Autodesk Inventor part; units mm, degrees
ref_plane "Work Plane1" through (150, 0, 0) normal (1, 0, 0) x (0, 0, -1)
ref_plane "Work Plane2" through (100.659, 0, -74) normal (0, 0, -1) x (-1, 0, 0)
ref_plane "Work Plane3" through (150, 0, 0) normal (1, 0, 0) x (0, 0, -1)
sketch "Sketch1" plane through (0, 0, 0) normal (0, 1, 0) x (-1, 0, 0)
  line L0 (0, 0) -> (-300, 0)
  line L1 (-300, 0) -> (-300, -148)
  line L2 (-300, -148) -> (0, -148)
  line L3 (0, -148) -> (0, 0)
  dimension "d0" = 300
  dimension "d1" = 148
extrude "Extrusion1" add sketch "Sketch1" along normal blind 4
sketch "Sketch2" plane through (0, 0, 0) normal (0, -1, 0) x (1, 0, 0)
  line L0 (0, -74) -> (300, -74) construction
  line L1 (150, 0) -> (150, -148) construction
sketch "Sketch3" plane through (0, 0, 0) normal (0, -1, 0) x (1, 0, 0)
  line L0 (0, -148) -> (70, -148)
  line L1 (70, -148) -> (70, -125)
  line L2 (70, -125) -> (0, -125)
  line L3 (0, -125) -> (0, -148)
  point P0 (0, 0)
  dimension "d4" = 70
  dimension "d5" = 23
extrude "Extrusion2" cut sketch "Sketch3" against normal blind 10
fillet "Fillet1" radius 10 1 edges at (0, 2, -125)
sketch "Sketch4" plane through (0, 0, 0) normal (0, -1, 0) x (1, 0, 0)
  line L0 (70, -125) -> (100.659, -148)
  line L1 (300, -148) -> (70, -148)
  line L2 (70, -148) -> (70, -125)
  line L3 (70, -125) -> (70, -148)
  point P0 (0, 0)
extrude "Extrusion3" cut sketch "Sketch4" against normal blind 10
ref_plane "Work Plane1" through (150, 0, 0) normal (1, 0, 0) x (0, 0, -1)
ref_plane "Work Plane2" through (100.659, 0, -74) normal (0, 0, -1) x (-1, 0, 0)
mirror "Mirror2" about plane through (100.659, 0, -74) normal (0, 0, -1) of "Extrusion2", "Extrusion3"
fillet "Fillet2" radius 10 1 edges at (0, 2, -23)
sketch "Sketch6" plane through (0, 0, 0) normal (0, -1, 0) x (1, 0, 0)
  point P0 (0, 0)
ref_plane "Work Plane3" through (150, 0, 0) normal (1, 0, 0) x (0, 0, -1)
mirror "Mirror3" about plane through (150, 0, 0) normal (1, 0, 0) of "Extrusion2", "Extrusion3", "Mirror2"
chamfer "Chamfer1" distance 8 angle 45 2 edges at (300, 2, -23) (300, 2, -125)
fillet "Fillet3" radius 8 4 edges at (199.341, 2, 0) (100.659, 2, 0) (199.341, 2, -148) (100.659, 2, -148)
sketch "Sketch7" plane through (0, 4, 0) normal (0, 1, 0) x (1, 0, 0)
  point P0 (0, 0)
properties part number "Basetrimed" material "ABS Plastic"
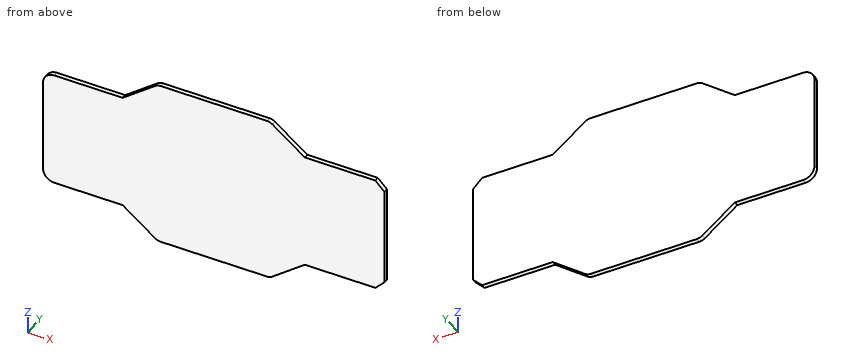
For this review, take the finished solid that the model builds, in its own axes (mm). Give positions to 0.01 mm unless a question says otherwise; leave off trailing zeros. Write each loop counter-clockwise with the first axis right and the second up, starting at its lowest first coordinate (ties: lowest second). Pieces come first, ordered by that corner, then holes. Notation, with made-up numbers: M -37,-21.75 L -12,-21.75 A34 cw -12,11.25 Z; hole C 24.5,66.5 d7. An arc over 180 degrees is marked long. One line per item, written item: value.
1) For line 1 (Z direction, x = 64, y = 2.95); line 2 (X direction, y = 3.1, z = -139); line 3 (Z direction, x = 228, y = 0.4), list the stretches that pass through material, from the lowest coordinate up. Write a range as from..to.
Results are:
line 1: z = -125..-23
line 2: x = 88.66..211.34
line 3: z = -126.5..-21.5
2) Take a section at A-A, the plane y = 1.55. Write out the cut boundary in (x, z).
Results are:
outline: M 0,-115 A10 ccw 10,-125 L 70,-125 L 98.53,-146.4 A8 ccw 103.33,-148 L 196.67,-148 A8 ccw 201.47,-146.4 L 230,-125 L 292,-125 L 300,-117 L 300,-31 L 292,-23 L 230,-23 L 201.47,-1.6 A8 ccw 196.67,0 L 103.33,0 A8 ccw 98.53,-1.6 L 70,-23 L 10,-23 A10 ccw 0,-33 Z
3) For P1, Ø1.5, axis at y = 2, z = -80, coming from the -X side, flat-tipped, find the tip position at first contact; note if it passes through.
Results are:
P1: stops at x = 0
4) Take a section at B-B, the plane x = 235.5. Write out the cut boundary in (y, z).
Results are:
outline: M 0,-125 L 4,-125 L 4,-23 L 0,-23 Z
5) Take a section at C-C, the plane z = -135. Write out the cut boundary in (x, y).
Results are:
outline: M 83.33,0 L 216.67,0 L 216.67,4 L 83.33,4 Z
